from build123d import *

# Parameters (mm, degrees)
SKETCH1_W           = 300
SKETCH1_H           = 400
SKETCH1_R           = 4
SKETCH1_R_2         = 4.5
BOSS_EXTRUDE1_DEPTH = 25


with BuildPart() as part:
    # Sketch1 → Boss-Extrude1 (new body)
    with BuildSketch(Plane.XY):
        Rectangle(SKETCH1_W, SKETCH1_H)
        with Locations((-112, -145)):
            Circle(SKETCH1_R, mode=Mode.SUBTRACT)
        with Locations((-140, -145)):
            Circle(SKETCH1_R, mode=Mode.SUBTRACT)
        with Locations(Location((112, -145, 0), (0, 0, 180))):
            Circle(SKETCH1_R, mode=Mode.SUBTRACT)
        with Locations(Location((140, -145, 0), (0, 0, 180))):
            Circle(SKETCH1_R, mode=Mode.SUBTRACT)
        with Locations((15, 145)):
            Circle(SKETCH1_R_2, mode=Mode.SUBTRACT)
        with Locations((-13, 145)):
            Circle(SKETCH1_R_2, mode=Mode.SUBTRACT)
        with Locations((27, 14)):
            Circle(SKETCH1_R_2, mode=Mode.SUBTRACT)
        with Locations((140, 45)):
            Circle(SKETCH1_R, mode=Mode.SUBTRACT)
        with Locations((112, 45)):
            Circle(SKETCH1_R, mode=Mode.SUBTRACT)
        with Locations(Location((-112, 45, 0), (0, 0, 180))):
            Circle(SKETCH1_R, mode=Mode.SUBTRACT)
        with Locations(Location((-140, 45, 0), (0, 0, 180))):
            Circle(SKETCH1_R, mode=Mode.SUBTRACT)
    extrude(amount=-BOSS_EXTRUDE1_DEPTH)


solid = part.part
Check sheet for the modelled part. Datum: model origin and axes. Units: mm. Round coordinates to 2 decimals unless told otherwise and drop trailing zeros. Loops run counter-clockwise (first coordinate to the right, second up) from the corner with the lowest first, then second, coordinate; pieces in that order, holes last. Notation, with made-up numbers: (7.5, 53.5) - (39.5, 53.5) arc R11 ccw to (39.5, 60.5) - close; hole circle Ø9 at (37, 3.25). An arc over 180 degrees is marked (long way). Answer as CSV lines item,"result". Start each with the question number.
Item 1: Release check for a two-part mould opening along Y. For faces 1 (the flat face through (-2, 3, 0)), 2 (the cylindrical face through (137.85, -148.373, -12.325)), 3 (the flat face through (-2, 200, -12)) record: +Y half, -Y half, draft (parallel to the pull), parting line (faces both ways), or undercut.
Item 2: Section check B-B (y = 14). Record the boundary of the cut face in (x, z), and give its area (4 significant figures).
Item 3: Section check A-A (x = 27). Record the boundary of the cut face in (y, z), and give its area (4 significant figures).
Item 4: Scan lines: line 1 (Y direction, x = 140, z = -14); line 2 (Y direction, x = 137, z = -14); line 3 (Y direction, x = 15, z = -11.25). Record each from-to range of solid material in increasing order. Write a range as [from, to].
Report:
1,face 1,"draft"
1,face 2,"undercut"
1,face 3,"+Y half"
2,outline,"(-150, -25) - (22.5, -25) - (22.5, 0) - (-150, 0) - close; (31.5, -25) - (150, -25) - (150, 0) - (31.5, 0) - close"
2,area,"7,275 mm2"
3,outline,"(-200, -25) - (9.5, -25) - (9.5, 0) - (-200, 0) - close; (18.5, -25) - (200, -25) - (200, 0) - (18.5, 0) - close"
3,area,"9,775 mm2"
4,line 1,"y = [-200, -149], [-141, 41], [49, 200]"
4,line 2,"y = [-200, -147.65], [-142.35, 42.35], [47.65, 200]"
4,line 3,"y = [-200, 140.5], [149.5, 200]"
